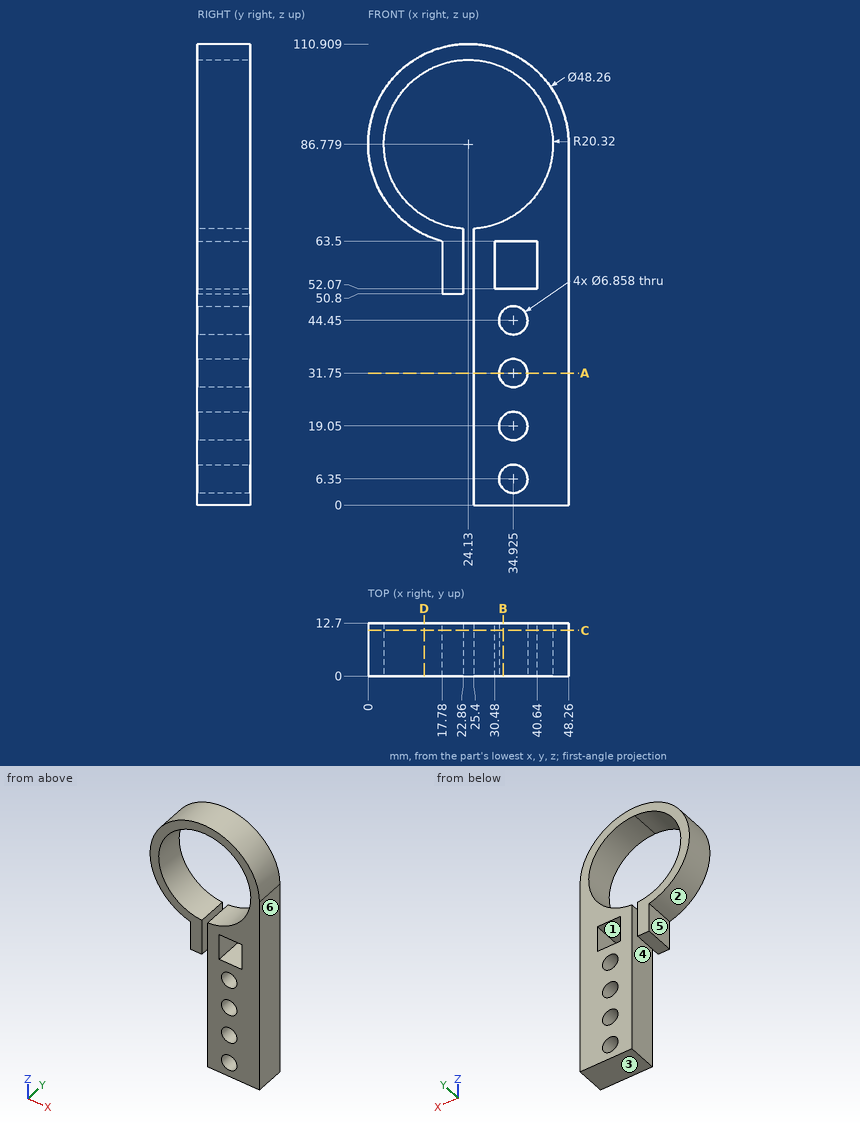
Geometry: see drawing. Coordinates: mm, zero at the bounding-box minimum. A direction names the side the tool comes from. Coordinates: 2 decimals unless noted, no trailing zeros. Loops run counter-clockwise (first coordinate to the right, second up) from the corner with the lowest first, then second, coordinate; pieces in that order, holes last. Notation, with made-up numbers: (11, 30.25) - (50, 30.25) arc R12 cw to (50, 35.25) - close; hole circle Ø8 at (65, 65.25). An arc over 180 degrees is marked (long way). Put each result on its own line as item: value. Start each with the question number.
Q1. Cut plane D-D, the plane x = 13.5. Return loops of the section in (y, z), and give its area (3 significant figures).
Q2. Cut plane B-B, the plane x = 32.5. Return loops of the section in (y, z) (1 decimal).
Q3. Cut plane A-A, the plane z = 31.75. Return loops of the section in (x, y), and give its area (3 significant figures).
Q4. Cut plane C-C, the plane y = 11. Give the number of separate pieces and of enclosed holes in the cut face, and give its area (3 significant figures).
Q5. Set-up query: the marked faces 4, 5 and 6. Return all of +Z, -Z, +X, -X, +Y, -Y with unobstructed straight access to the full face (end or side cutting, diameter ignored); none if empty.
Q6. Pull-direction query (Z, two-part tool) for the marked faces 1, 2 and 3; classes: released by +Z, released by -Z, zero draft, split by the parting line, or undercut.
Q7. Line query: line 1 (X direction, y = 5.75, z = 44.45); line 2 (X direction, y = 5.25, z = 62); line 3 (Z direction, x = 39, y = 6.5) (1 decimal). Output: solid intervals per line, ascending.
Q8. Pin query (flat end, axial travel): pin 1 Ø1 at (x, y) = (5.5, 7.5) entering from +Z (1 decimal); pin 2 Ø9 at (x, z) = (34.925, 31.75) entering from -Y; pin 3 Ø6.5 at (y, z) = (8, 54.5) entering from -X; pin 4 Ø2 at (x, y) = (17, 10) entering from -Z. Return the tip coordinate at first contact, or that it passes through.
Filled sheet:
1. outline: (0, 65.12) - (12.7, 65.12) - (12.7, 69.46) - (0, 69.46) - close; (0, 104.1) - (12.7, 104.1) - (12.7, 108.44) - (0, 108.44) - close
1. area: 110 mm²
2. outline: (0, 0) - (12.7, 0) - (12.7, 3.9) - (0, 3.9) - close; (0, 8.8) - (12.7, 8.8) - (12.7, 16.6) - (0, 16.6) - close; (0, 21.5) - (12.7, 21.5) - (12.7, 29.3) - (0, 29.3) - close; (0, 34.2) - (12.7, 34.2) - (12.7, 42) - (0, 42) - close; (0, 46.9) - (12.7, 46.9) - (12.7, 52.1) - (0, 52.1) - close; (0, 63.5) - (12.7, 63.5) - (12.7, 68.3) - (0, 68.3) - close; (0, 105.3) - (12.7, 105.3) - (12.7, 109.4) - (0, 109.4) - close
3. outline: (25.4, 0) - (31.5, 0) - (31.5, 12.7) - (25.4, 12.7) - close; (38.35, 0) - (48.26, 0) - (48.26, 12.7) - (38.35, 12.7) - close
3. area: 203 mm²
4. separate pieces: 1
4. enclosed holes: 5
4. area: 1,880 mm²
5. face 4: -Z, +Y, -Y
5. face 5: -Z, -X, +Y, -Y
5. face 6: +Z, -Z, +X, +Y, -Y
6. face 1: undercut
6. face 2: split by the parting line
6. face 3: released by -Z
7. line 1: 25.4 to 31.5, 38.35 to 48.26
7. line 2: 17.78 to 22.86, 25.4 to 30.48, 40.64 to 48.26
7. line 3: 0 to 52.1, 63.5 to 72.9, 100.6 to 105.8
8. pin 1: z = 102.7
8. pin 2: y = 0
8. pin 3: x = 17.78
8. pin 4: z = 50.8
